Read the model definition and answer for the solid it produces. Units are mm, in the model's axes. Face numbers are marked on the shaded views. A direction names the side the tool comes from. Give positions to 0.01 mm unless a question says otherwise; leave off trailing zeros. Write each loop counter-clockwise with the first axis right and the second up, starting at its lowest first coordinate (ties: lowest second). Pieces come first, ordered by that corner, then holes. Notation, with made-up numbers: M 53.25,6.25 L 71.25,6.25 A8 ccw 71.25,15.25 Z; hole C 31.25,15 d6. An arc over 180 degrees is marked long. Use a Markdown table: item, result. Add a question column.
Item 1: For the marked faces 1 and 2, determine the directions among +Z, -Z, +X, -X, +Y, -Y from which every point of the face is accessible in a straight line to the end or side of a thin tool.
Item 2: A cutting plane is placed at C-C on z = 2. Determine the outline of the cut face in (x, y), then the cut area to 3 significant figures.
Item 3: A cutting plane is placed at A-A on y = 0. Determine the outline of the cut face in (x, z), then the cut area to 3 significant figures.
Item 4: The mould has two halves that part along Y. Classify the marked faces 3, 4, 5 and 6: pulls with the +Y half, pulls with the -Y half, needs draft (parallel to the pull), parting line crosses it, or undercut.
Item 5: A cutting plane is placed at B-B on x = 0. Determine the outline of the cut face in (y, z).
Item 6: A cutting plane is placed at D-D on x = 5.25. Determine the outline of the cut face in (y, z).
Item 7: Consider probe 1 along X at (y, z) = (0.75, 4.5); probe 2 along X at (y, z) = (-1.25, 2); probe 3 along Y at (x, z) = (4.5, 6). Determine where each line is inside the solid, lowest interval first. Write a range as [from, to].
Item 8: Given P1, Ø2.5, axis at x = 8, z = 4, coming from the +Y side; P2, Ø2.5, axis at x = 7.5, z = 6, coming from the -Y side, each flat-ended and moving along its own axis, determine where each tip first touches the part or whether it passes through.
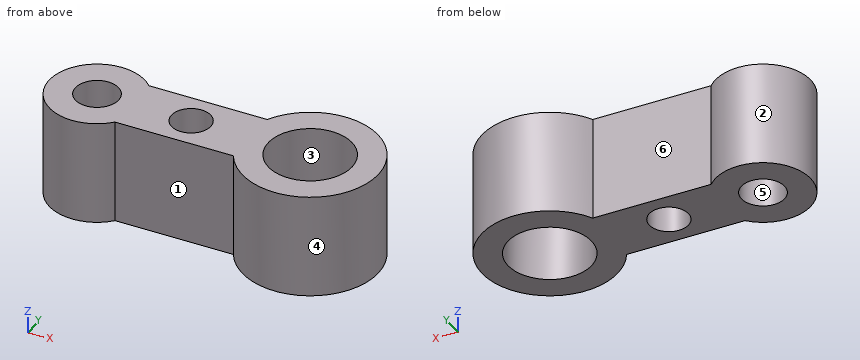
from build123d import *

# Parameters (mm, degrees)
CROQUIS1_R              = 3.2
CROQUIS1_R_2            = 1.65
SALIENTE_EXTRUIR1_DEPTH = 8
CROQUIS3_R              = 1.5
CORTAR_EXTRUIR1_DEPTH   = 21.5


with BuildPart() as part:
    # Croquis1 → Saliente-Extruir1 (new body)
    with BuildSketch(Plane.XY):
        with BuildLine():
            Line((11.659417229, 2.5), (2.659417229, 2.5))
            ThreePointArc((2.659417229, 2.5), (-3.65, 0), (2.659417229, -2.5))
            Line((2.659417229, -2.5), (11.659417229, -2.5))
            ThreePointArc((11.659417229, -2.5), (21.419022475, 0), (11.659417229, 2.5))
        make_face()
        with Locations((16.219022475, 0)):
            Circle(CROQUIS1_R, mode=Mode.SUBTRACT)
        Circle(CROQUIS1_R_2, mode=Mode.SUBTRACT)
    extrude(amount=SALIENTE_EXTRUIR1_DEPTH)

    # Croquis3 → Cortar-Extruir1 (cut)
    with BuildSketch(Plane(origin=(0, 0, 0), x_dir=(-1, 0, 0), z_dir=(0, 0, -1))):
        with Locations((-7.159417229, 0)):
            Circle(CROQUIS3_R)
    extrude(amount=-CORTAR_EXTRUIR1_DEPTH, mode=Mode.SUBTRACT)


solid = part.part
Filled in:
| question | item | result |
|---|---|---|
| 1 | face 1 | +Z, -Z, -Y |
| 1 | face 2 | +Z, -Z |
| 2 | outline | M 2.66,-2.5 L 11.66,-2.5 A5.2 ccw long 11.66,2.5 L 2.66,2.5 A3.65 ccw long Z; hole C 0,0 d3.3; hole C 7.16,0 d3; hole C 16.22,0 d6.4 |
| 2 | area | 118 mm² |
| 3 | outline | M -3.65,0 L -1.65,0 L -1.65,8 L -3.65,8 Z; M 1.65,0 L 5.66,0 L 5.66,8 L 1.65,8 Z; M 8.66,0 L 13.02,0 L 13.02,8 L 8.66,8 Z; M 19.42,0 L 21.42,0 L 21.42,8 L 19.42,8 Z |
| 3 | area | 99.0 mm² |
| 4 | face 3 | undercut |
| 4 | face 4 | parting line crosses it |
| 4 | face 5 | undercut |
| 4 | face 6 | pulls with the +Y half |
| 5 | outline | M -3.65,0 L -1.65,0 L -1.65,8 L -3.65,8 Z; M 1.65,0 L 3.65,0 L 3.65,8 L 1.65,8 Z |
| 6 | outline | M -2.5,0 L 2.5,0 L 2.5,8 L -2.5,8 Z |
| 7 | probe 1 | [-3.57, -1.47], [1.47, 5.86], [8.46, 13.11], [19.33, 21.36] |
| 7 | probe 2 | [-3.43, -1.08], [1.08, 6.33], [7.99, 13.27], [19.16, 21.27] |
| 7 | probe 3 | [-2.5, 2.5] |
| 8 | P1 | y = 2.5 |
| 8 | P2 | y = -2.5 |
